Autodesk Inventor part; units mm, degrees
ref_plane "YZ Plane" through (0, 0, 0) normal (1, 0, 0) x (0, 1, 0)
ref_plane "XZ Plane" through (0, 0, 0) normal (0, 1, 0) x (-1, 0, 0)
ref_plane "XY Plane" through (0, 0, 0) normal (0, 0, 1) x (1, 0, 0)
surface "Composite1"
sketch "Sketch2" plane through (0, -23.8125, 0) normal (0, 0, 1) x (1, 0, 0)
  arc A0 (3.8159, 50.4746) -> (21.182, 40.4482) centre (24.1677, 65.6722) ccw
  arc A1 (3.8159, 50.4746) -> (-3.8159, 50.4746) centre (0, 47.625) ccw
  arc A2 (-21.182, 40.4482) -> (-3.8159, 50.4746) centre (-24.1677, 65.6722) ccw
  arc A3 (-21.182, 40.4482) -> (-24.998, 33.8388) centre (-20.6222, 35.7187) ccw
  arc A4 (-24.998, 13.7862) -> (-24.998, 33.8388) centre (-48.3354, 23.8125) ccw
  arc A5 (-24.998, 13.7862) -> (-21.182, 7.1768) centre (-20.6222, 11.9062) ccw
  arc A6 (-3.8159, -2.8496) -> (-21.182, 7.1768) centre (-24.1677, -18.0472) ccw
  arc A7 (-3.8159, -2.8496) -> (3.8159, -2.8496) centre (0, 0) ccw
  arc A8 (21.182, 7.1768) -> (3.8159, -2.8496) centre (24.1677, -18.0472) ccw
  arc A9 (21.182, 7.1768) -> (24.998, 13.7862) centre (20.6222, 11.9063) ccw
  arc A10 (24.998, 33.8388) -> (24.998, 13.7862) centre (48.3354, 23.8125) ccw
  arc A11 (24.998, 33.8388) -> (21.182, 40.4482) centre (20.6222, 35.7188) ccw
  circle A12 centre (0, 47.625) radius 1.7272
  circle A13 centre (20.6222, 35.7188) radius 1.7272
  circle A14 centre (20.6222, 11.9063) radius 1.7272
  circle A15 centre (0, 0) radius 1.7272
  circle A16 centre (-20.6222, 11.9062) radius 1.7272
  circle A17 centre (-20.6222, 35.7187) radius 1.7272
  arc A18 (14.2875, 23.8125) -> (-14.2875, 23.8125) centre (0, 23.8125) ccw
  arc A19 (-14.2875, 23.8125) -> (14.2875, 23.8125) centre (0, 23.8125) ccw
  circle A20 centre (0, 23.8125) radius 12.7
extrude "Extrusion1" add sketch "Sketch2" along normal blind 6.35 contours A0 A11 A10 A9 A8 A7 A6 A5 A4 A3 A2 A1
extrude "Extrusion2" add sketch "Sketch2" along normal blind 3.175 contours A19 A18
sketch "Sketch3" plane through (0, -23.8125, 6.35) normal (0, 0, 1) x (1, 0, 0)
  circle A0 centre (0, 23.8125) radius 14.2875
  circle A1 centre (0, 23.8125) radius 15.875
  circle A2 centre (0, 23.8125) radius 12.7
  dimension "d4" = 31.75
extrude "Extrusion3" cut sketch "Sketch3" against normal blind 3.175 contours A1
extrude "Extrusion4" cut sketch "Sketch3" against normal through all contours A0
chamfer "Chamfer1" distance 2.9972 angle 45 6 edges at (18.895, 11.9063, 0) (-1.7272, 23.8125, 0) (-22.3494, 11.9063, 0) (-22.3494, -11.9062, 0) (-1.7272, -23.8125, 0) (18.895, -11.9062, 0)
properties part number "lower box bolt plate"
Check sheet for the modelled part. Datum: model origin and axes. Units: mm. A direction names the side the tool comes from. Round coordinates to 2 decimals unless told otherwise and drop trailing zeros. Loops run counter-clockwise (first coordinate to the right, second up) from the corner with the lowest first, then second, coordinate; pieces in that order, holes last. Notation, with made-up numbers: (67.25, 1) - (93.25, 1) arc R29 cw to (93.25, 23) - close; hole circle Ø11 at (-4.5, 27). An arc over 180 degrees is marked (long way). Write item = value, one per line. Start each with the question number.
Q1. Access from +Z, -Z, +X, -X, +Y, -Y to the whole of each face (thin tool, end or side, straight path). Record for faces 4 (the face through (-11.83, 8.31, 3.175)), 5 (the face through (-0.225, -25.525, 4.65)).
Q2. Section check D-D (z = 2). Record the boundary of the cut face in (x, y) (1 decimal), plus the area to 3 significant figures.
Q3. Thickness scan on L1, parallel to X at y = 12, z = 5.25; L2, parallel to Y at x = 0.5, z = 1.5; L3, parallel to Y at x = -18.5, z = 0.75. Record the ranges inside material, lowest first.
Q4. Release check for a two-part mould opening along X. For faces 1 (the face through (-19.74, -10.21, 2.81)), 2 (the face through (11.593, 19.791, 3.131)), 3 (the face through (-24.78, 14.23, 3.13)) record: pulls with the +X half, pulls with the -X half, needs draft (parallel to the pull), parting line crosses it, or undercut.
Q5. Section check C-C (x = -8.5). Record the boundary of the cut face in (y, z) (3 decimals).
Q6. Section check B-B (x = 0). Count the separate pieces of the cut face and the enclosed holes in it, plus the area to 3 significant figures.
Q7. Depth check by flat-ended pin: P1, Ø4.5, axis at x = 20.62, y = 11.91, coming from the -Z side; P2, Ø4, axis at x = -20.62, y = -11.91, coming from the -Z side. Enter the tip coordinate at first touch or a pass-through.
Derived:
q1.face_4 = +Z
q1.face_5 = +Z, -Z
q2.outline = (-25, -10) arc R4.8 ccw to (-21.2, -16.6) arc R25.4 cw to (-3.8, -26.7) arc R4.8 ccw to (3.8, -26.7) arc R25.4 cw to (21.2, -16.6) arc R4.8 ccw to (25, -10) arc R25.4 cw to (25, 10) arc R4.8 ccw to (21.2, 16.6) arc R25.4 cw to (3.8, 26.7) arc R4.8 ccw to (-3.8, 26.7) arc R25.4 cw to (-21.2, 16.6) arc R4.8 ccw to (-25, 10) arc R25.4 cw to start; hole circle Ø5.4 at (-20.6, -11.9); hole circle Ø5.4 at (-20.6, 11.9); hole circle Ø28.6 at (0, 0); hole circle Ø5.4 at (0, -23.8); hole circle Ø5.4 at (0, 23.8); hole circle Ø5.4 at (20.6, -11.9); hole circle Ø5.4 at (20.6, 11.9)
q2.area = 1,230 mm^2
q3.L1 = -25.38 to -22.35, -18.9 to -10.39, 10.39 to 18.9, 22.35 to 25.38
q3.L2 = -28.55 to -27, -20.63 to -14.28, 14.28 to 20.63, 27 to 28.55
q3.L3 = -17.1 to -15.27, -8.55 to 8.55, 15.27 to 17.1
q4.face_1 = undercut
q4.face_2 = pulls with the +X half
q4.face_3 = pulls with the -X half
q5.outline = (-21.868, 0) - (-11.484, 0) - (-11.484, 3.175) - (-13.408, 3.175) - (-13.408, 6.35) - (-21.868, 6.35) - close; (11.484, 0) - (21.868, 0) - (21.868, 6.35) - (13.408, 6.35) - (13.408, 3.175) - (11.484, 3.175) - close
q6.separate_pieces = 4
q6.enclosed_holes = 0
q6.area = 110 mm^2
q7.P1 = 2.47
q7.P2 = 2.72
